For this review, use the dimensioned drawing (mm, ordinates from the lowest corner) and the shaded views. A direction names the side the tool comes from. Give positions to 0.01 mm unless a question says otherwise; leave off trailing zeros. Order: outer loops, then holes, each group sorted by start corner. A loop starts at its lowest first (then second) coordinate and runs counter-clockwise, first axis right, second up. Notation, with made-up numbers: (32.5, -20.75) -> (55.5, -20.75) arc R16 ccw to (55.5, -7.75) -> close; hole circle Ø10 at (-8, 28.25). An arc over 180 degrees is marked (long way). Answer as a JSON object with one key per item and string values. Group by question number.
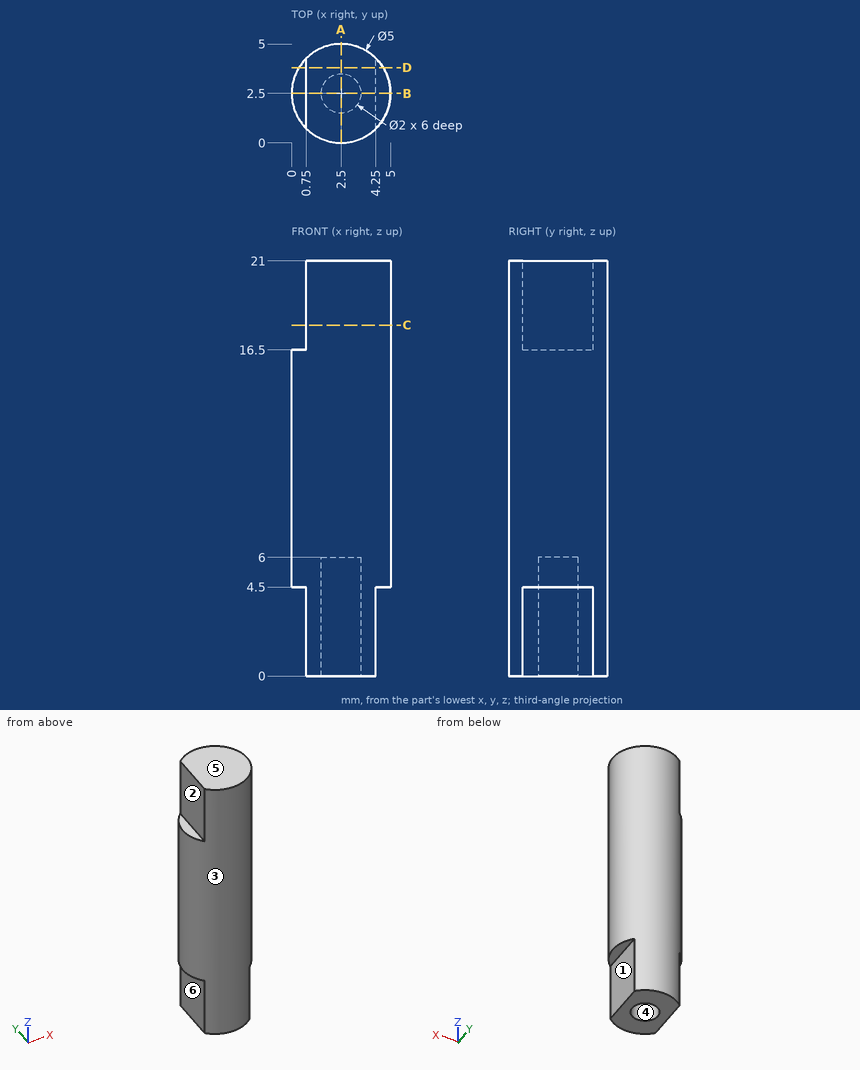
1. Machinability: for the marked faces 1, 2 and 3, which of the approach directions +Z, -Z, +X, -X, +Y, -Y give a long, thin tool a straight path to every point of the face, cutting with its end or side? Answer none if there is none.
2. Take a section at B-B on y = 2.5. Give the boundary of the cut face in (x, z).
3. Take a section at D-D on y = 3.8. Give the boundary of the cut face in (x, z).
4. For probe 1 along Y at (x, z) = (2.5, 2); probe 2 along Z at (x, y) = (4.6, 3.8); probe 3 along Z at (x, y) = (3, 1.8), list the stretches that pass through material, from the lowest coordinate up. Write a range as [from, to].
5. For pin 1 (1.2 mm diameter, centred on x = 2.5, y = 2.5, fed in from -Z); pin 2 (1.5 mm diameter, centred on y = 1.5, z = 11, fed in from -X), all flat-tipped, find the tip position at first contact; note any pin that passes through.
6. Draft analysis for pull direction X (two halves, no side actions). For the marked faces 4, 5 and 6, state which applies: pulls with the +X half, pulls with the -X half, needs draft (parallel to the pull), parting line crosses it, or undercut.
7. Take a section at A-A on x = 2.5. Give the boundary of the cut face in (y, z).
8. Take a section at C-C on z = 17.75. Give the boundary of the cut face in (x, y), plus the area to 3 significant figures.
Checks:
{
 "1": {"face 1": "-Z, +X, +Y, -Y", "face 2": "+Z, -X, +Y, -Y", "face 3": "+Z, -Z"},
 "2": {"outline": "(0, 4.5) -> (0.75, 4.5) -> (0.75, 0) -> (1.5, 0) -> (1.5, 6) -> (3.5, 6) -> (3.5, 0) -> (4.25, 0) -> (4.25, 4.5) -> (5, 4.5) -> (5, 21) -> (0.75, 21) -> (0.75, 16.5) -> (0, 16.5) -> close"},
 "3": {"outline": "(0.36, 4.5) -> (0.75, 4.5) -> (0.75, 0) -> (4.25, 0) -> (4.25, 4.5) -> (4.64, 4.5) -> (4.64, 21) -> (0.75, 21) -> (0.75, 16.5) -> (0.36, 16.5) -> close"},
 "4": {"probe 1": "y = [0, 1.5], [3.5, 5]", "probe 2": "z = [4.5, 21]", "probe 3": "z = [6, 21]"},
 "5": {"pin 1": "stops at z = 6", "pin 2": "stops at x = 0.01"},
 "6": {"face 4": "undercut", "face 5": "needs draft", "face 6": "pulls with the -X half"},
 "7": {"outline": "(0, 0) -> (1.5, 0) -> (1.5, 6) -> (3.5, 6) -> (3.5, 0) -> (5, 0) -> (5, 21) -> (0, 21) -> close"},
 "8": {"outline": "(0.75, 0.71) arc R2.5 ccw (long way) to (0.75, 4.29) -> close", "area": "17.8 mm2"}
}
